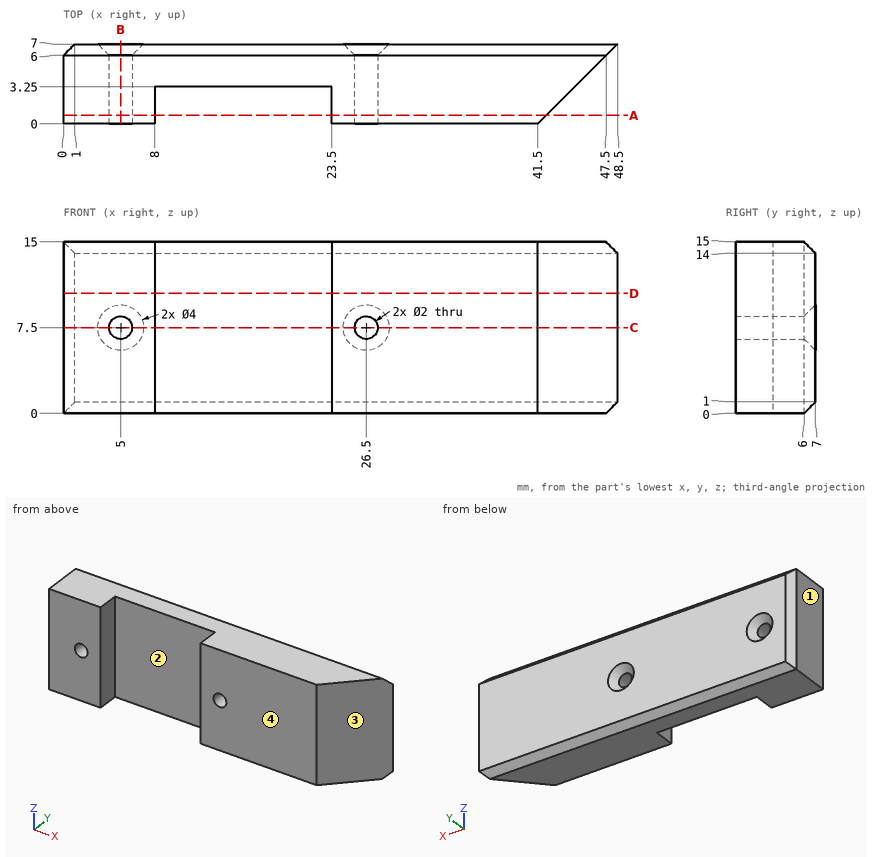
Answer from the drawing. Dimensions are ordinates in mm from the lowest x, y and z of the part. Give positions to 0.01 mm unless a question says otherwise; leave off trailing zeros. Order: outer loops, then holes, each group sorted by start corner. A loop starts at its lowest first (then second) coordinate and runs counter-clockwise, first axis right, second up.
(1) Find section B-B (x = 5). Give the vertices of the cut face in (y, z).
(2) For a pull along X with two mould halves and no side action, classify the marked faces 1, 2, 3 and 4 as released by +X, released by -X, zero draft, split by the parting line, or undercut.
(3) Find section D-D (z = 10.5). Give the vertices of the cut face in (x, y), plus the area to 3 significant figures.
(4) Find section C-C (z = 7.5). Give the vertices of the cut face in (x, y).
(5) Given pin 1 (3 mm diameter, centred on y = 4.5, z = 8, fed in from +X); pin 2 (1 mm diameter, centred on y = 5, z = 12.5, fed in from +X); pin 3 (2.5 mm diameter, centred on x = 5, z = 7.5, fed in from +Y), each flat-ended and moving along its own axis, determine where each tip first touches the part or whether it passes through.
(6) Find section A-A (y = 0.75). Give the vertices of the cut face in (x, z).
(7) Straight lines are drawn through the part: L1, parallel to Z at x = 26.5, y = 4; L2, parallel to Y at x = 23, z = 7.5; L3, parallel to X at y = 1.5, z = 13. For each, find the intervals that lie inside material, in ascending order.
Result sheet:
1. outline: (0, 0) - (6, 0) - (7, 1) - (7, 5.5) - (6, 6.5) - (0, 6.5) - close; (0, 8.5) - (6, 8.5) - (7, 9.5) - (7, 14) - (6, 15) - (0, 15) - close
2. face 1: released by -X
2. face 2: undercut
2. face 3: released by +X
2. face 4: zero draft
3. outline: (0, 0) - (8, 0) - (8, 3.25) - (23.5, 3.25) - (23.5, 0) - (41.5, 0) - (48.5, 7) - (1, 7) - (0, 6) - close
3. area: 264 mm2
4. outline: (0, 0) - (4, 0) - (4, 6) - (3, 7) - (1, 7) - (0, 6) - close; (6, 0) - (8, 0) - (8, 3.25) - (23.5, 3.25) - (23.5, 0) - (25.5, 0) - (25.5, 6) - (24.5, 7) - (7, 7) - (6, 6) - close; (27.5, 0) - (41.5, 0) - (48.5, 7) - (28.5, 7) - (27.5, 6) - close
5. pin 1: stops at x = 47.5
5. pin 2: stops at x = 47
5. pin 3: stops at y = 6.25
6. outline: (0, 0) - (8, 0) - (8, 15) - (0, 15) - close; (23.5, 0) - (42.25, 0) - (42.25, 15) - (23.5, 15) - close; hole circle Ø2 at (5, 7.5); hole circle Ø2 at (26.5, 7.5)
7. L1: z = 0 to 6.5, 8.5 to 15
7. L2: y = 3.25 to 7
7. L3: x = 0 to 8, 23.5 to 43
